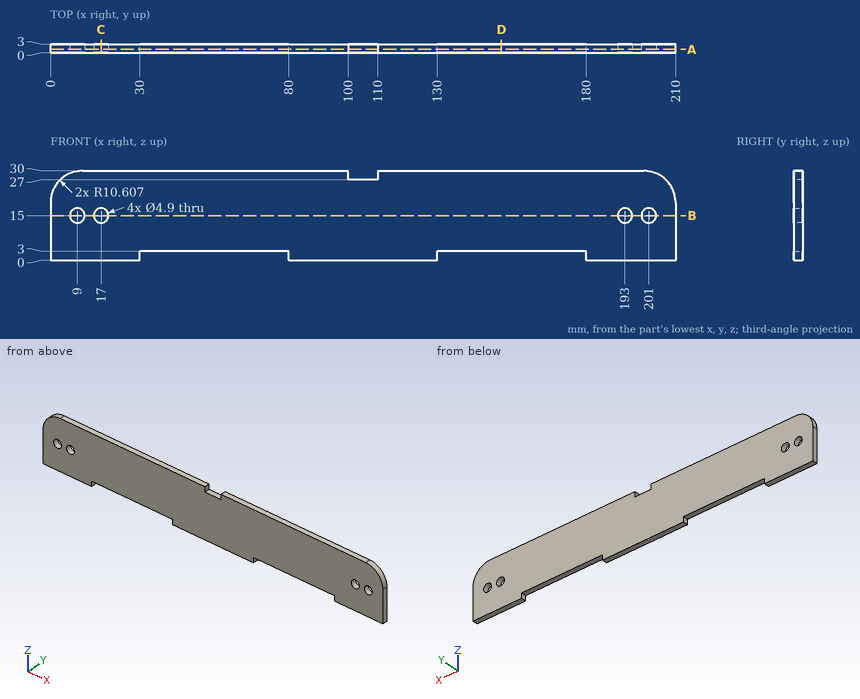
Part print with two shaded views. Sizes in mm from the minimum x, y, z corner. Give positions to 0.01 mm unless a question says otherwise; leave off trailing zeros. Order: outer loops, then holes, each group sorted by start corner. A loop starts at its lowest first (then second) coordinate and runs counter-clockwise, first axis right, second up.
(1) Drill centre lines: L1, parallel to X at y = 0.8, z = 15; L2, parallel to Z at x = 17, y = 1.1; L3, parallel to X at y = 0.7, z = 13 (1 decimal). Where is each one in solid material? Low to high.
(2) Saw through at D-D, the plane x = 151.5. Give the cut face in (y, z).
(3) Saw through at A-A, the plane y = 1.2. Give the cut face in (x, z).
(4) Flat gauge pins, fed straight in: pin 1 (3 mm diameter, centred on x = 9, z = 15, fed in from +Y); pin 2 (4 mm diameter, centred on x = 69.5, z = 4.5, fed in from -Y); pin 3 (0.9 mm diameter, centred on x = 47.5, y = 2, fed in from -Z); pin 4 (1.5 mm diameter, centred on y = 1, z = 29, fed in from +X). Where does each tip first touch, or does it go through?
(5) Saw through at C-C, the plane x = 17. Give the cut face in (y, z), then the cut area to 3 significant figures.
(6) Saw through at B-B, the plane z = 15. Give the cut face in (x, y).
Results found:
1. L1: x = 0 to 6.55, 11.45 to 14.55, 19.45 to 190.55, 195.45 to 198.55, 203.45 to 210
1. L2: z = 0 to 12.55, 17.45 to 30
1. L3: x = 0 to 7.6, 10.4 to 15.6, 18.4 to 191.6, 194.4 to 199.6, 202.4 to 210
2. outline: (0, 3) - (3, 3) - (3, 30) - (0, 30) - close
3. outline: (0, 0) - (30, 0) - (30, 3) - (80, 3) - (80, 0) - (130, 0) - (130, 3) - (180, 3) - (180, 0) - (210, 0) - (210, 19.39) arc R10.61 ccw to (199.39, 30) - (110, 30) - (110, 27) - (100, 27) - (100, 30) - (10.61, 30) arc R10.61 ccw to (0, 19.39) - close; hole circle Ø4.9 at (9, 15); hole circle Ø4.9 at (17, 15); hole circle Ø4.9 at (193, 15); hole circle Ø4.9 at (201, 15)
4. pin 1: passes through
4. pin 2: stops at y = 0
4. pin 3: stops at z = 3
4. pin 4: stops at x = 205.23
5. outline: (0, 0) - (3, 0) - (3, 12.55) - (0, 12.55) - close; (0, 17.45) - (3, 17.45) - (3, 30) - (0, 30) - close
5. area: 75.3 mm2
6. outline: (0, 0) - (6.55, 0) - (6.55, 3) - (0, 3) - close; (11.45, 0) - (14.55, 0) - (14.55, 3) - (11.45, 3) - close; (19.45, 0) - (190.55, 0) - (190.55, 3) - (19.45, 3) - close; (195.45, 0) - (198.55, 0) - (198.55, 3) - (195.45, 3) - close; (203.45, 0) - (210, 0) - (210, 3) - (203.45, 3) - close
